from build123d import *

# Parameters (mm, degrees)
F0_W     = 15
F0_H     = 15
F0_R     = 5
F1_DEPTH = 15
F3_DEPTH = 15.001
F5_DEPTH = 15.001
F6_R     = 1


with BuildPart() as f1:
    # F0 (on Top) → F1 (new body)
    with BuildSketch(Plane.XY):
        with Locations((7.5, 7.5)):
            Rectangle(F0_W, F0_H)
        with Locations((7.5, 7.5)):
            Circle(F0_R, mode=Mode.SUBTRACT)
    extrude(amount=F1_DEPTH)

    # F2 (on face) → F3 (cut, through all)
    with BuildSketch(Plane.XZ):
        with BuildLine():
            Line((2.5, 7.5), (12.5, 7.5))
            ThreePointArc((12.5, 7.5), (7.5, 12.5), (2.5, 7.5))
        make_face()
        with BuildLine():
            ThreePointArc((2.5, 7.5), (7.5, 2.5), (12.5, 7.5))
            Line((12.5, 7.5), (2.5, 7.5))
        make_face()
    extrude(amount=-F3_DEPTH, mode=Mode.SUBTRACT)

    # F4 (on face) → F5 (cut, through all)
    with BuildSketch(Plane(origin=(0, 0, 0), x_dir=(0, -1, 0), z_dir=(-1, 0, 0))):
        with BuildLine():
            Line((-12.5, 7.5), (-2.5, 7.5))
            ThreePointArc((-2.5, 7.5), (-7.5, 12.5), (-12.5, 7.5))
        make_face()
        with BuildLine():
            ThreePointArc((-12.5, 7.5), (-7.5, 2.5), (-2.5, 7.5))
            Line((-2.5, 7.5), (-12.5, 7.5))
        make_face()
    extrude(amount=-F5_DEPTH, mode=Mode.SUBTRACT)

    # F6
    f6_edges = [f1.edges().sort_by_distance(p)[0] for p in [
        (0, 7.5, 15),
        (7.5, 0, 15),
        (0, 0, 7.5),
        (15, 0, 7.5),
        (7.5, 0, 0),
        (0, 7.5, 0),
        (0, 15, 7.5),
        (7.5, 15, 15),
        (15, 7.5, 15),
        (15, 7.5, 0),
        (15, 15, 7.5),
        (7.5, 15, 0),
    ]]
    fillet(f6_edges, radius=F6_R)


solid = f1.part
For this review, take the finished solid that the model builds, in its own axes (mm). Round coordinates to 2 decimals unless told otherwise and drop trailing zeros. Loops run counter-clockwise (first coordinate to the right, second up) from the corner with the lowest first, then second, coordinate; pieces in that order, holes last. Notation, with made-up numbers: (-34.75, -28.75) - (-0.75, -28.75) arc R27 cw to (-0.75, -8.75) - close; hole circle Ø11 at (26.25, -19). An arc over 180 degrees is marked (long way). Use one line per item in the form item = value.
1) Wall thickness on probe 1 along Y at (x, z) = (7.5, 13.9): over which ranges is the line inside the solid? List them lowest first.
Solutions:
probe_1 = 0 to 2.5, 12.5 to 15
2) We need section C-C on x = 3.5. Write out the cut boundary in (y, z).
Solutions:
outline = (0, 1) arc R1 ccw to (1, 0) - (4.5, 0) - (4.5, 3.5) arc R5 cw to (3.5, 4.5) - (0, 4.5) - close; (0, 10.5) - (3.5, 10.5) arc R5 cw to (4.5, 11.5) - (4.5, 15) - (1, 15) arc R1 ccw to (0, 14) - close; (10.5, 0) - (14, 0) arc R1 ccw to (15, 1) - (15, 4.5) - (11.5, 4.5) arc R5 cw to (10.5, 3.5) - close; (10.5, 11.5) arc R5 cw to (11.5, 10.5) - (15, 10.5) - (15, 14) arc R1 ccw to (14, 15) - (10.5, 15) - close
3) We need section A-A on z = 7.5. Write out the cut boundary in (x, y), then the cut area to 3 significant figures.
Solutions:
outline = (0, 1) arc R1 ccw to (1, 0) - (2.5, 0) - (2.5, 2.5) - (0, 2.5) - close; (0, 12.5) - (2.5, 12.5) - (2.5, 15) - (1, 15) arc R1 ccw to (0, 14) - close; (12.5, 0) - (14, 0) arc R1 ccw to (15, 1) - (15, 2.5) - (12.5, 2.5) - close; (12.5, 12.5) - (15, 12.5) - (15, 14) arc R1 ccw to (14, 15) - (12.5, 15) - close
area = 24.1 mm2
4) Mouldability with a two-part tool opening along Y and no side actions: class faces 1 (the face through (0.285, 7.591, 14.699)), 2 (the face through (13.431, 2.505, 7.28)), 3 (the face through (4.5, 15, 3.1)), 4 (the face through (1.514, 3.815, 4.121)) as pulls with the +Y half, pulls with the -Y half, needs draft (parallel to the pull), parting line crosses it, or undercut.
Solutions:
face_1 = needs draft
face_2 = undercut
face_3 = pulls with the +Y half
face_4 = undercut
5) Clearance check with a flat-ended pin moving along its axis: P1, Ø6, axis at y = 7.5, z = 7.5, coming from the -X side. State where the tip first meets the part, or that it passes through.
Solutions:
P1 = through
6) We need section D-D on y = 13.5. Write out the cut boundary in (x, z).
Solutions:
outline = (0, 1) arc R1 ccw to (1, 0) - (14, 0) arc R1 ccw to (15, 1) - (15, 14) arc R1 ccw to (14, 15) - (1, 15) arc R1 ccw to (0, 14) - close; hole circle Ø10 at (7.5, 7.5)
